Part model, mm, in its own coordinate system. A direction names the side the tool comes from. Coordinates: 2 decimals unless noted, no trailing zeros. Write each loop counter-clockwise with the first axis right and the second up, starting at its lowest first coordinate (ties: lowest second). Pieces come first, ordered by that corner, then holes. Notation, with made-up numbers: (-14.5, -31.5) -> (24.5, -31.5) arc R17 ccw to (24.5, -14.5) -> close; hole circle Ø1 at (77.5, -15). An arc over 180 degrees is marked (long way). One line per question, with ' | ' between items. Start each with the question number.
Item 1: 3-axis set-ups, long thin cutter, end or side, ignore diameter. For faces 1 (the flat face through (23, -6.35, 21)), 2 (the flat face through (23, -13, 17.984)), 3 (the flat face through (117, -13, 14.174)): which of +Z, -Z, +X, -X, +Y, -Y reach the whole face in a straight line?
Item 2: Probe probe 1 along X at (y, z) = (-8.5, 15.25); probe 2 along X at (y, z) = (-3.75, 13.25); probe 3 along Z at (x, y) = (46, -19.5). List the from-to ranges inside material, lowest first. Write a range as [from, to].
Item 3: Two-plate mould, pull along Z, no slides. Class faces 4 (the cylindrical face through (68.828, -12.878, 15.514)), 5 (the cylindrical face through (88.629, -12.593, 27.535)), 6 (the flat face through (25.964, -13, 17)): pulls with the +Z half, pulls with the -Z half, needs draft (parallel to the pull), parting line crosses it, or undercut.
Item 4: Saw through at A-A (y = -11.25). List the corners of the cut face in (x, z) (1 decimal), and give its area (3 significant figures).
Item 5: Pin check, flat tips, straight feed: pin 1 (1.5 mm diameter, centred on x = 106, y = -22, fed in from -Z); pin 2 (5 mm diameter, centred on x = 53, z = 24, fed in from +Y); pin 3 (14 mm diameter, centred on x = 118.5, y = -9, fed in from -Z); pin 4 (3 mm diameter, centred on x = 105.5, y = -15, fed in from -Z). Stop position of each tip, or through.
from build123d import *

# Parameters (mm, degrees)
F1_DEPTH = 12.7
F2_R     = 2.54
F3_DEPTH = 12.7
F4_SCALE = 2
F5_W     = 12.7
F5_H     = 6.35
F6_DEPTH = 6.35
F7_R     = 1.5875
F8_DEPTH = 25.4


with BuildPart() as f1:
    # F0 (on Front) → F1 (new body)
    with BuildSketch(Plane.XZ):
        with BuildLine():
            Line((61.5102246263, 7.086984636), (61.5102246263, 7.848984636))
            ThreePointArc((61.5102246263, 7.848984636), (44.0614550619, 13.8211347469), (25.6817610527, 15.341984636))
            Line((25.6817610527, 15.341984636), (25.6817610527, 5.816984636))
            ThreePointArc((25.6817610527, 5.816984636), (40.4209928395, 6.5545750011), (55.1602246263, 5.816984636))
            Line((55.1602246263, 5.816984636), (55.1602246263, 7.086984636))
            Line((55.1602246263, 7.086984636), (61.5102246263, 7.086984636))
        make_face()
    extrude(amount=F1_DEPTH)

    # F2
    f2_edges = [f1.edges().sort_by_distance(p)[0] for p in [
        (44.061455, -12.7, 13.821135),
        (44.061455, 0, 13.821135),
    ]]
    fillet(f2_edges, radius=F2_R)

    # F3 (add): a face of the model
    f3_faces = [f1.faces().sort_by_distance(p)[0] for p in [
        (25.6817610527, -6.35, 10.4811297922),
    ]]
    extrude(f3_faces, amount=F3_DEPTH)


with BuildPart() as f1_1:
    # F4: moved
    add(f1.part.scale(F4_SCALE))

    # F5 (on face) → F6 (join)
    with BuildSketch(Plane(origin=(25.9635221053, 0, 0), x_dir=(0, -1, 0), z_dir=(-1, 0, 0))):
        with Locations((12.7, 21.1589692719)):
            Rectangle(F5_W, F5_H)
    extrude(amount=F6_DEPTH)

    # F7 (on face) → F8 (cut)
    with BuildSketch(Plane.XZ.offset(25.4)):
        with Locations((70.4135221053, 15.4439692719)):
            Circle(F7_R)
    extrude(amount=-F8_DEPTH, mode=Mode.SUBTRACT)


solid = f1_1.part
From the geometry:
1) face 1: +Z, -Z, -X, +Y | face 2: -Z, -X, +Y, -Y | face 3: -Z, +X, +Y, -Y
2) probe 1: [25.96, 68.84], [71.99, 123.02] | probe 2: [25.96, 110.32] | probe 3: [11.63, 30.68]
3) face 4: undercut | face 5: pulls with the +Z half | face 6: needs draft
4) outline: (19.6, 18) -> (26, 18) -> (26, 11.6) -> (51.4, 11.6) arc R295.3 cw to (110.3, 11.6) -> (110.3, 14.2) -> (123, 14.2) -> (123, 15.7) arc R149.6 ccw to (51.4, 30.7) -> (26, 30.7) -> (26, 24.3) -> (19.6, 24.3) -> close; hole circle Ø3.2 at (70.4, 15.4) | area: 1,480 mm2
5) pin 1: z = 11.97 | pin 2: y = 0 | pin 3: z = 14.17 | pin 4: z = 11.95
